Work out the finished part from the listing and answer in its coordinate system (mm). A direction names the side the tool comes from. Coordinates: 2 decimals unless noted, no trailing zeros. One line per question, with ' | ' between items.
```python
from build123d import *

# Parameters (mm, degrees)
BOSS_EXTRUDE1_DEPTH             = 304.8
SKETCH2_R                       = 5.55625
CUT_EXTRUDE1_DEPTH              = 304.8
SKETCH3_R                       = 5.55625
CUT_EXTRUDE2_DEPTH              = 304.8
SKETCH4_W                       = 57.15
SKETCH4_H                       = 304.8
CUT_EXTRUDE3_DEPTH              = 4
SWEEP1_PROFILE_R                = 15.875
BOSS_EXTRUDE2_REACH             = 426.804
BOSS_EXTRUDE2_END_RADIUS        = 15.875
SKETCH18_R                      = 15.875
BOSS_EXTRUDE2_DIRECTION_2_DEPTH = 25.4


with BuildPart() as part:
    # Sketch1 → Boss-Extrude1 (new body)
    with BuildSketch(Plane(origin=(0, 0, 0), x_dir=(1, 0, 0), z_dir=(0, 1, 0))):
        with BuildLine():
            Line((2, 0), (55.15, 0))
            ThreePointArc((55.15, 0), (56.564213562, 0.585786438), (57.15, 2))
            Line((57.15, 2), (57.15, 55.15))
            ThreePointArc((57.15, 55.15), (56.564213562, 56.564213562), (55.15, 57.15))
            Line((55.15, 57.15), (2, 57.15))
            ThreePointArc((2, 57.15), (0.585786438, 56.564213562), (0, 55.15))
            Line((0, 55.15), (0, 2))
            ThreePointArc((0, 2), (0.585786438, 0.585786438), (2, 0))
        make_face()
        with BuildLine():
            Line((4.667, 54.483), (52.483, 54.483))
            ThreePointArc((52.483, 54.483), (53.897213562, 53.897213562), (54.483, 52.483))
            Line((54.483, 52.483), (54.483, 4.667))
            ThreePointArc((54.483, 4.667), (53.897213562, 3.252786438), (52.483, 2.667))
            Line((52.483, 2.667), (4.667, 2.667))
            ThreePointArc((4.667, 2.667), (3.252786438, 3.252786438), (2.667, 4.667))
            Line((2.667, 4.667), (2.667, 52.483))
            ThreePointArc((2.667, 52.483), (3.252786438, 53.897213562), (4.667, 54.483))
        make_face(mode=Mode.SUBTRACT)
    extrude(amount=BOSS_EXTRUDE1_DEPTH)

    # Sketch2 → Cut-Extrude1 (cut)
    with BuildSketch(Plane.XY):
        with Locations((28.575, 292.1)):
            Circle(SKETCH2_R)
        with Locations((28.575, 266.7)):
            Circle(SKETCH2_R)
        with Locations((28.575, 241.3)):
            Circle(SKETCH2_R)
        with Locations((28.575, 215.9)):
            Circle(SKETCH2_R)
        with Locations((28.575, 190.5)):
            Circle(SKETCH2_R)
        with Locations((28.575, 165.1)):
            Circle(SKETCH2_R)
        with Locations((28.575, 139.7)):
            Circle(SKETCH2_R)
        with Locations((28.575, 114.3)):
            Circle(SKETCH2_R)
        with Locations((28.575, 88.9)):
            Circle(SKETCH2_R)
        with Locations((28.575, 63.5)):
            Circle(SKETCH2_R)
        with Locations((28.575, 38.1)):
            Circle(SKETCH2_R)
        with Locations((28.575, 12.7)):
            Circle(SKETCH2_R)
    extrude(amount=-CUT_EXTRUDE1_DEPTH, mode=Mode.SUBTRACT)

    # Sketch3 → Cut-Extrude2 (cut)
    with BuildSketch(Plane(origin=(57.15, 0, -57.15), x_dir=(0, 0, 1), z_dir=(-1, 0, 0))):
        with Locations(Location((28.575, 292.1, 0), (0, 0, 180))):
            Circle(SKETCH3_R)
        with Locations(Location((28.575, 266.7, 0), (0, 0, 180))):
            Circle(SKETCH3_R)
        with Locations(Location((28.575, 241.3, 0), (0, 0, 180))):
            Circle(SKETCH3_R)
        with Locations(Location((28.575, 215.9, 0), (0, 0, 180))):
            Circle(SKETCH3_R)
        with Locations(Location((28.575, 190.5, 0), (0, 0, 180))):
            Circle(SKETCH3_R)
        with Locations(Location((28.575, 165.1, 0), (0, 0, 180))):
            Circle(SKETCH3_R)
        with Locations(Location((28.575, 139.7, 0), (0, 0, 180))):
            Circle(SKETCH3_R)
        with Locations(Location((28.575, 114.3, 0), (0, 0, 180))):
            Circle(SKETCH3_R)
        with Locations(Location((28.575, 88.9, 0), (0, 0, 180))):
            Circle(SKETCH3_R)
        with Locations(Location((28.575, 63.5, 0), (0, 0, 180))):
            Circle(SKETCH3_R)
        with Locations(Location((28.575, 38.1, 0), (0, 0, 180))):
            Circle(SKETCH3_R)
        with Locations(Location((28.575, 12.7, 0), (0, 0, 180))):
            Circle(SKETCH3_R)
    extrude(amount=CUT_EXTRUDE2_DEPTH, mode=Mode.SUBTRACT)

    # Sketch4 → Cut-Extrude3 (cut)
    with BuildSketch(Plane(origin=(0, 0, -57.15), x_dir=(-1, 0, 0), z_dir=(0, 0, -1))):
        with Locations((-28.575, 152.4)):
            Rectangle(SKETCH4_W, SKETCH4_H)
    extrude(amount=-CUT_EXTRUDE3_DEPTH, mode=Mode.SUBTRACT)

    # Sweep1: sweep along a path in Sketch5
    with BuildLine(Plane(origin=(28.575, 0, 0), x_dir=(0, 0, -1), z_dir=(1, 0, 0))) as sweep1_path:
        Line((2, 25.4), (-252, 25.4))
        Line((-252, 25.4), (2, 279.4))
        Line((2, 279.4), (10.980256121, 288.380256121))
    # Sweep1 profile (on start of the path) → Sweep1 (sweep)
    with BuildSketch(Plane(origin=(28.575, 25.4, -2), x_dir=(1, 0, 0), z_dir=(0, 0, 1))):
        Circle(SWEEP1_PROFILE_R)
    sweep(path=sweep1_path.line, transition=Transition.RIGHT)

    # Boss-Extrude2: up to this cylinder (the profile starts outside it)
    boss_extrude2_end = Plane(origin=(28.575, 25.4, 252), z_dir=(0, 0, -1)) * Cylinder(BOSS_EXTRUDE2_END_RADIUS, 886.358, mode=Mode.PRIVATE)
    # Sketch18 → Boss-Extrude2 (add, up to the surface)
    with BuildSketch(Plane(origin=(0, 0, 0), x_dir=(1, 0, 0), z_dir=(0, 1, 0)), mode=Mode.PRIVATE) as boss_extrude2_sk1:
        with Locations(Location((28.575, -252, 0), (0, 0, 270))):
            Circle(SKETCH18_R)
    boss_extrude2_tool1 = extrude(boss_extrude2_sk1.sketch, amount=BOSS_EXTRUDE2_REACH, mode=Mode.PRIVATE) - boss_extrude2_end
    add(boss_extrude2_tool1.solids().sort_by_distance((28.575, 0, 252))[0])

    # Sketch18 → Boss-Extrude2 direction 2 (add)
    with BuildSketch(Plane(origin=(0, 0, 0), x_dir=(1, 0, 0), z_dir=(0, 1, 0))):
        with Locations(Location((28.575, -252, 0), (0, 0, 270))):
            Circle(SKETCH18_R)
    extrude(amount=-BOSS_EXTRUDE2_DIRECTION_2_DEPTH)

    # Sketch19 → Revolve1 (revolve)
    with BuildSketch(Plane(origin=(28.575, 0, 0), x_dir=(0, 0, -1), z_dir=(1, 0, 0)), mode=Mode.PRIVATE) as revolve1_sk:
        Polygon((-236.125, -25.4), (-236.125, -50.8), (-213.9, -76.2), (-252, -76.2), (-252, -25.4), align=None)
    revolve(revolve1_sk.sketch.rotate(Axis((28.575, -25.4, 252), (0, -1, 0)), 180), axis=Axis((28.575, -25.4, 252), (0, -1, 0)))


solid = part.part
```
1) Find the intervals of material crossed by line 1 along X through (y, z) = (165, -2); line 2 along Z through (x, y) = (2, 88); line 3 along Z through (x, y) = (55, 108), in increasing order.
Check values:
line 1: x = 0 to 23.02, 34.13 to 57.15 | line 2: z = -53.15 to -34.06, -23.09 to 0 | line 3: z = -53.15 to 0
2) The mould has two halves that part along X. Classify faces 1 (the face through (35.9, 11.316, 126.778)), 2 (the face through (1.352, 170.524, -27.371)), 3 (the face through (31.562, 169.785, -1.315)): released by +X, released by -X, zero draft, split by the parting line, or undercut.
Check values:
face 1: split by the parting line | face 2: zero draft | face 3: undercut
3) For faces 4 (the face through (29.11, 269.65, -14.69)), 5 (the face through (28, 14, -2)), 6 (the face through (28.459, 9.525, 271.252)), 7 (the face through (1.352, 135.015, -31.562)), determine the directions among +Z, -Z, +X, -X, +Y, -Y from which every point of the face is accessible in a straight line to the end or side of a thin tool.
Check values:
face 4: none | face 5: -Z | face 6: +Z | face 7: +X, -X
4) Flat-ended cylindrical pins translate along their axes: pin 1 (13 mm diameter, centred on x = 28.575, y = 241.3, fed in from +Z); pin 2 (4 mm diameter, centred on x = 36.5, z = 158.5, fed in from -Y); pin 3 (18 mm diameter, centred on x = 28.575, y = 88.9, fed in from +Z). Find the tip coordinate at first contact, or state that the pin passes through.
Check values:
pin 1: stops at z = 65.05 | pin 2: stops at y = 10.67 | pin 3: stops at z = 219.95
5) Find section A-A (y = 165.1). State how many separate pieces and enclosed holes the cut face has, plus the area to 3 significant figures.
Check values:
separate pieces: 5 | enclosed holes: 0 | area: 1,450 mm^2
